Could you check a few things on this drawing? It's one solid part, dimensions in mm from its lowest x, y, z. A direction names the side the tool comes from. Give positions to 0.01 mm unless a question says otherwise; leave off trailing zeros. Order: outer loops, then holes, each group sorted by start corner. A loop starts at its lowest first (then second) coordinate and runs counter-clockwise, first axis right, second up.
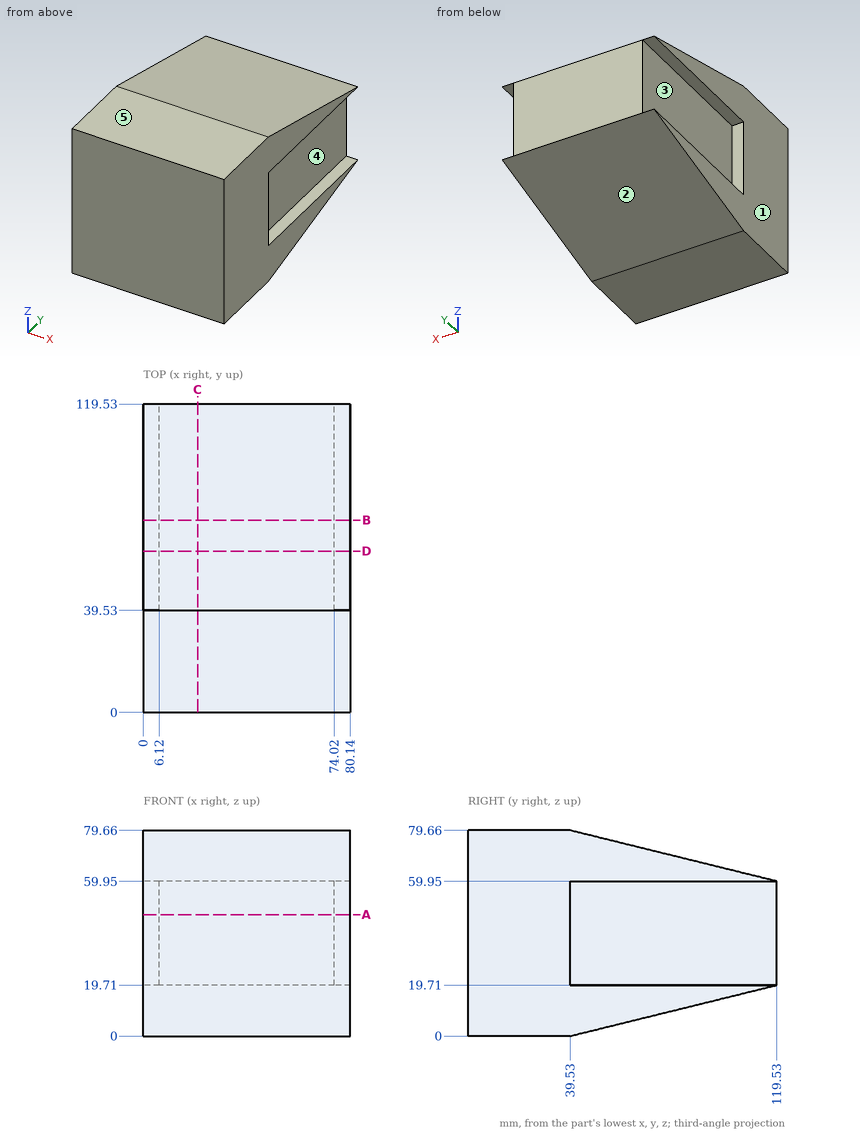
Item 1: Imagine slicing it at A-A on z = 47. List the corners of the cut face in (x, y) for me.
Findings:
outline: (0, 0) - (80.14, 0) - (80.14, 39.53) - (74.02, 39.53) - (74.02, 119.53) - (6.12, 119.53) - (6.12, 39.53) - (0, 39.53) - close
Item 2: Imagine slicing it at C-C on x = 21. List the corners of the cut face in (y, z) for me, then the cut area to 3 significant figures.
Findings:
outline: (0, 0) - (39.53, 0) - (119.53, 19.71) - (119.53, 59.95) - (39.53, 79.66) - (0, 79.66) - close
area: 7,940 mm2
Item 3: For the marked faces 4 and 5, which set-ups out of +Z, -Z, +X, -X, +Y, -Y let a thin tool reach every point of the face, with its end or its side?
Findings:
face 4: +X, +Y
face 5: +Z, +X, -X, +Y, -Y
Item 4: Imagine slicing it at D-D on y = 62.5. List the corners of the cut face in (x, z) for me, then the cut area to 3 significant figures.
Findings:
outline: (0, 5.66) - (80.14, 5.66) - (80.14, 19.71) - (74.02, 19.71) - (74.02, 59.95) - (80.14, 59.95) - (80.14, 74) - (0, 74) - (0, 59.95) - (6.12, 59.95) - (6.12, 19.71) - (0, 19.71) - close
area: 4,980 mm2
Item 5: Imagine slicing it at B-B on y = 74.5. List the corners of the cut face in (x, z) for me, then the cut area to 3 significant figures.
Findings:
outline: (0, 8.62) - (80.14, 8.62) - (80.14, 19.71) - (74.02, 19.71) - (74.02, 59.95) - (80.14, 59.95) - (80.14, 71.04) - (0, 71.04) - (0, 59.95) - (6.12, 59.95) - (6.12, 19.71) - (0, 19.71) - close
area: 4,510 mm2
Item 6: We'd pull the mould along Z, two halves only. Please class the marked faces 1, 2 and 3: +Z half, -Z half, draft (parallel to the pull), parting line (faces both ways), or undercut.
Findings:
face 1: draft
face 2: -Z half
face 3: undercut
Item 7: Please list where these lines run through material, in increasing order: line 1 along Z through (x, y) = (76.5, 86.5); line 2 along X through (y, z) = (84, 31); line 3 along Z through (x, y) = (5.5, 62).
Findings:
line 1: z = 11.57 to 19.71, 59.95 to 68.09
line 2: x = 6.12 to 74.02
line 3: z = 5.54 to 19.71, 59.95 to 74.12
Item 8: For pin 1 (12 mm diameter, centred on y = 86, z = 35.5, fed in from -X); pin 2 (12 mm diameter, centred on x = 60, z = 43, fed in from -Y); pin 3 (8 mm diameter, centred on x = 66, y = 92.5, fed in from +Z) (3 decimals); pin 4 (4 mm diameter, centred on x = 31.5, y = 52.5, fed in from -Z), each with a flat end and sliding along its axis, tell me the tip position at first contact or that it passes through.
Findings:
pin 1: stops at x = 6.12
pin 2: stops at y = 0
pin 3: stops at z = 67.595
pin 4: stops at z = 2.7
